```python
from build123d import *

# Parameters (mm, degrees)
SALIENTE_EXTRUIR1_DEPTH = 8.5
CROQUIS2_R              = 1.25
CORTAR_EXTRUIR1_DEPTH   = 8.5
CROQUIS3_R              = 3
CORTAR_EXTRUIR2_DEPTH   = 2.5


with BuildPart() as part:
    # Croquis1 → Saliente-Extruir1 (new body)
    with BuildSketch(Plane.XY):
        Polygon((12.15, 8.15), (12.15, 5.65), (10.15, 6.275), (10.15, -6.275), (12.15, -5.65), (12.15, -8.15), (10.15, -7.525), (10.15, -10.15), (15.165647838, -10.15), (15.165647838, 10.15), (10.15, 10.15), (10.15, 7.525), align=None)
    extrude(amount=SALIENTE_EXTRUIR1_DEPTH)

    # Croquis2 → Cortar-Extruir1 (cut)
    with BuildSketch(Plane.ZY.offset(-10.15)):
        with Locations((4.25, 0)):
            Circle(CROQUIS2_R)
    extrude(amount=-CORTAR_EXTRUIR1_DEPTH, mode=Mode.SUBTRACT)

    # Croquis3 → Cortar-Extruir2 (cut)
    with BuildSketch(Plane.ZY.offset(-10.15)):
        with Locations((4.25, 0)):
            Circle(CROQUIS3_R)
    extrude(amount=-CORTAR_EXTRUIR2_DEPTH, mode=Mode.SUBTRACT)


solid = part.part
```
Work out the finished part from the listing and answer in its coordinate system (mm). A direction names the side the tool comes from. Give positions to 0.01 mm unless a question says otherwise; leave off trailing zeros. Write each loop counter-clockwise with the first axis right and the second up, starting at its lowest first coordinate (ties: lowest second). Pieces come first, ordered by that corner, then holes.
(1) The part is cut by section B-B on x = 10.75. Write down the section's boundary in (y, z), plus the area to 3 significant figures.
Final values:
outline: (-10.15, 0) - (-7.71, 0) - (-7.71, 8.5) - (-10.15, 8.5) - close; (-6.09, 0) - (6.09, 0) - (6.09, 8.5) - (-6.09, 8.5) - close; (7.71, 0) - (10.15, 0) - (10.15, 8.5) - (7.71, 8.5) - close; hole circle Ø6 at (0, 4.25)
area: 117 mm2
(2) The part is cut by section C-C on z = 4.25. Write down the section's boundary in (x, y) (3 decimals).
Final values:
outline: (10.15, -10.15) - (15.166, -10.15) - (15.166, -1.25) - (12.65, -1.25) - (12.65, -3) - (10.15, -3) - (10.15, -6.275) - (12.15, -5.65) - (12.15, -8.15) - (10.15, -7.525) - close; (10.15, 3) - (12.65, 3) - (12.65, 1.25) - (15.166, 1.25) - (15.166, 10.15) - (10.15, 10.15) - (10.15, 7.525) - (12.15, 8.15) - (12.15, 5.65) - (10.15, 6.275) - close
(3) The part is cut by section A-A on y = 0. Write down the section's boundary in (x, z), plus the area to 3 significant figures.
Final values:
outline: (10.15, 0) - (15.17, 0) - (15.17, 3) - (12.65, 3) - (12.65, 1.25) - (10.15, 1.25) - close; (10.15, 7.25) - (12.65, 7.25) - (12.65, 5.5) - (15.17, 5.5) - (15.17, 8.5) - (10.15, 8.5) - close
area: 21.3 mm2
(4) Straight lines are drawn through the part: line 1 (Y direction, x = 13.55, z = 4.25); line 2 (Y direction, x = 11, z = 6.5); line 3 (Y direction, x = 10.6, z = 1.75). For each, find the intervals that lie inside material, in ascending order.
Final values:
line 1: y = -10.15 to -1.25, 1.25 to 10.15
line 2: y = -10.15 to -7.79, -6.01 to -1.98, 1.98 to 6.01, 7.79 to 10.15
line 3: y = -10.15 to -7.67, -6.13 to -1.66, 1.66 to 6.13, 7.67 to 10.15
(5) Which of the six approach directions +Z, -Z, +X, -X, +Y, -Y give full straight-line access (tool end or side, diameter ignored) to faces 4 (the flat face through (12.65, 0, 6)), 5 (the flat face through (13, -10.15, 4)), 6 (the flat face through (11.16, -7.84, 4.19))?
Final values:
face 4: -X
face 5: +Z, -Z, +X, -X, -Y
face 6: +Z, -Z
(6) The part is cut by section D-D on z = 7.5. Write down the section's boundary in (x, y) (3 decimals).
Final values:
outline: (10.15, -10.15) - (15.166, -10.15) - (15.166, 10.15) - (10.15, 10.15) - (10.15, 7.525) - (12.15, 8.15) - (12.15, 5.65) - (10.15, 6.275) - (10.15, -6.275) - (12.15, -5.65) - (12.15, -8.15) - (10.15, -7.525) - close
(7) The mould has two halves that part along X. Classify faces 1 (the cylindrical face through (13.89, 0.38, 5.44)), 2 (the flat face through (12.15, -7, 4)), 3 (the flat face through (10.15, 9, 4)): pulls with the +X half, pulls with the -X half, needs draft (parallel to the pull), parting line crosses it, or undercut.
Final values:
face 1: needs draft
face 2: undercut
face 3: pulls with the -X half
(8) A flat-ended cylindrical pin translates along its axis: pin 1 Ø3 at (y, z) = (0, 5.5) entering from -X. Find the tip coordinate at first contact, or state that the pin passes through.
Final values:
pin 1: stops at x = 12.65
